```python
from build123d import *

# Parameters (mm, degrees)
SZKIC1_R                    = 5
SZKIC1_R_2                  = 4
DODANIE_WYCI_GNI_CIE1_DEPTH = 145
SZKIC2_R                    = 2.605682129
SZKIC2_R_2                  = 2.5
WYTNIJ_WYCI_GNI_CIE1_DEPTH  = 15


with BuildPart() as part:
    # Szkic1 → Dodanie-wyciągnięcie1 (new body)
    with BuildSketch(Plane(origin=(0, 0, 0), x_dir=(1, 0, 0), z_dir=(0, 1, 0))):
        Circle(SZKIC1_R)
        Circle(SZKIC1_R_2, mode=Mode.SUBTRACT)
    extrude(amount=DODANIE_WYCI_GNI_CIE1_DEPTH)

    # Szkic2 → Wytnij-wyciągnięcie1 (cut, symmetric)
    with BuildSketch(Plane.XY):
        with Locations((0, 140)):
            Circle(SZKIC2_R)
        with Locations((1.33e-07, 25)):
            Circle(SZKIC2_R_2)
    extrude(amount=WYTNIJ_WYCI_GNI_CIE1_DEPTH, both=True, mode=Mode.SUBTRACT)


solid = part.part
```
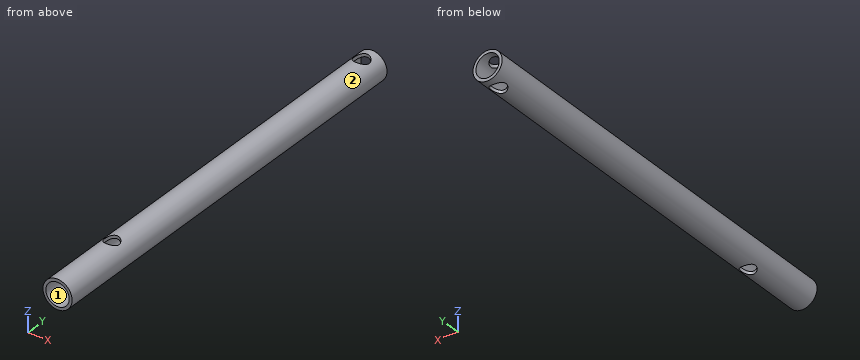
Model file for the job. Use its own axes, mm. Face numbers are marked on the shaded views. Coordinates: 2 decimals unless noted, no trailing zeros. Write each loop counter-clockwise with the first axis right and the second up, starting at its lowest first coordinate (ties: lowest second). Pieces come first, ordered by that corner, then holes. Notation, with made-up numbers: (-16, 55) - (-7, 55) arc R24 cw to (-7, 72) - close; hole circle Ø9 at (-1.5, 45). An arc over 180 degrees is marked (long way). Use a Markdown table: item, result. Add a question column.
Item 1: Band-saw the part on D-D, the plane y = 130.5. Write the cut outline in (x, z).
Item 2: Drill centre lines: line 1 along Y through (x, z) = (0, -4.45); line 2 along X through (y, z) = (45, -0.25). Where is each one in solid material? Low to high.
Item 3: Band-saw the part on C-C, the plane y = 25. Write the cut outline in (x, z).
Item 4: Two-plate mould, pull along X, no slides. Class the marked faces 1 and 2: pulls with the +X half, pulls with the -X half, needs draft (parallel to the pull), parting line crosses it, or undercut.
Item 5: Band-saw the part on A-A, the plane z = 0. Write the cut outline in (x, y), and give its area (3 significant figures).
Item 6: Band-saw the part on B-B, the plane x = 1. Write the cut outline in (y, z).
Item 7: Drop flat-ended pins along their axis: pin 1 (5 mm diameter, centred on x = -2, z = 2.5, fed in from -Y); pin 2 (1 mm diameter, centred on x = 2, y = 91.5, fed in from -Z); pin 3 (1 mm diameter, centred on x = 3.5, y = 86.5, fed in from -Z); pin 4 (2 mm diameter, centred on y = 106.5, z = -2.5, fed in from -X). Give the stop position or say it passes through.
A:
| question | item | result |
|---|---|---|
| 1 | outline | circle Ø10 at (0, 0); hole circle Ø8 at (0, 0) |
| 2 | line 1 | y = 0 to 22.5, 27.5 to 137.39, 142.61 to 145 |
| 2 | line 2 | x = -4.99 to -3.99, 3.99 to 4.99 |
| 3 | outline | (-2.5, -4.33) - (-2.5, -3.12) arc R4 cw to (-2.5, 3.12) - (-2.5, 4.33) arc R5 ccw to start; (2.5, -4.33) arc R5 ccw to (2.5, 4.33) - (2.5, 3.12) arc R4 cw to (2.5, -3.12) - close |
| 4 | face 1 | undercut |
| 4 | face 2 | parting line crosses it |
| 5 | outline | (-5, 0) - (-4, 0) - (-4, 145) - (-5, 145) - close; (4, 0) - (5, 0) - (5, 145) - (4, 145) - close |
| 5 | area | 290 mm² |
| 6 | outline | (0, -4.9) - (22.71, -4.9) - (22.71, -3.87) - (0, -3.87) - close; (0, 3.87) - (22.71, 3.87) - (22.71, 4.9) - (0, 4.9) - close; (27.29, -4.9) - (137.59, -4.9) - (137.59, -3.87) - (27.29, -3.87) - close; (27.29, 3.87) - (137.59, 3.87) - (137.59, 4.9) - (27.29, 4.9) - close; (142.41, -4.9) - (145, -4.9) - (145, -3.87) - (142.41, -3.87) - close; (142.41, 3.87) - (145, 3.87) - (145, 4.9) - (142.41, 4.9) - close |
| 7 | pin 1 | stops at y = 0 |
| 7 | pin 2 | stops at z = -4.77 |
| 7 | pin 3 | stops at z = -4 |
| 7 | pin 4 | stops at x = -4.77 |
